Autodesk Inventor part; units mm, degrees
ref_plane "YZ Plane" through (0, 0, 0) normal (1, 0, 0) x (0, 1, 0)
ref_plane "XZ Plane" through (0, 0, 0) normal (0, 1, 0) x (-1, 0, 0)
ref_plane "XY Plane" through (0, 0, 0) normal (0, 0, 1) x (1, 0, 0)
sketch "スケッチ1" plane through (0, 0, 0) normal (0, 0, 1) x (1, 0, 0)
  circle A0 centre (0, 0) radius 2.75
  dimension "d0" = 5.5
extrude "押し出し1" add sketch "スケッチ1" along normal blind 2
fillet "フィレット1" radius 1 1 edges at (-2.75, 0, 2)
sketch "スケッチ2" plane through (0, 0, 0) normal (0, 0, -1) x (-1, 0, 0)
  circle A0 centre (0, 0) radius 1.5
  dimension "d4" = 3
extrude "押し出し2" add sketch "スケッチ2" along normal blind 10
thread "ねじ1"
properties part number "Screw_10mm" material "真鍮"
Could you check a few things on this model? Use its own coordinates, in mm. A direction names the side the tool comes from. Coordinates: 2 decimals unless noted, no trailing zeros. Write each loop counter-clockwise with the first axis right and the second up, starting at its lowest first coordinate (ties: lowest second). Pieces come first, ordered by that corner, then holes. Notation, with made-up numbers: (59, 86.5) - (69, 86.5) arc R18 ccw to (69, 93.5) - close; hole circle Ø1 at (82, -37.75). An arc over 180 degrees is marked (long way). Write item = value, one per line.
1) Will this pin go through, and if not, where does the flat tip stop? pin 1 Ø1.5 at (x, z) = (-2, -2) entering from -Y.
Result set:
pin_1 = -0.83
2) Please list where these lines run through material, in increasing order: line 1 (Z direction, x = 2.2, y = 0); line 2 (Z direction, x = -2.1, y = -1.65); line 3 (X direction, y = -0.8, z = -2). Write a range as [from, to].
Result set:
line_1 = [0, 1.89]
line_2 = [0, 1.39]
line_3 = [-1.27, 1.27]
3) Suppose I cut it at D-D on z = 1.75. Please give me the cut outline in (x, y).
Result set:
outline = circle Ø4.82 at (0, 0)
4) Suppose I cut it at C-C on z = -1.5. Please give me the cut outline in (x, y).
Result set:
outline = circle Ø3 at (0, 0)
5) For faces 1 (the flat face through (0, 0, -10)), 2 (the cylindrical face through (1.5, -0.07, -4.93)), which set-ups out of +Z, -Z, +X, -X, +Y, -Y let a thin tool reach every point of the face, with its end or its side?
Result set:
face_1 = -Z, +X, -X, +Y, -Y
face_2 = -Z
6) Suppose I cut it at A-A on y = 0. Please give me the cut outline in (x, z), plus the area to 3 significant figures.
Result set:
outline = (-2.75, 0) - (-1.5, 0) - (-1.5, -10) - (1.5, -10) - (1.5, 0) - (2.75, 0) - (2.75, 1) arc R1 ccw to (1.75, 2) - (-1.75, 2) arc R1 ccw to (-2.75, 1) - close
area = 40.6 mm2
